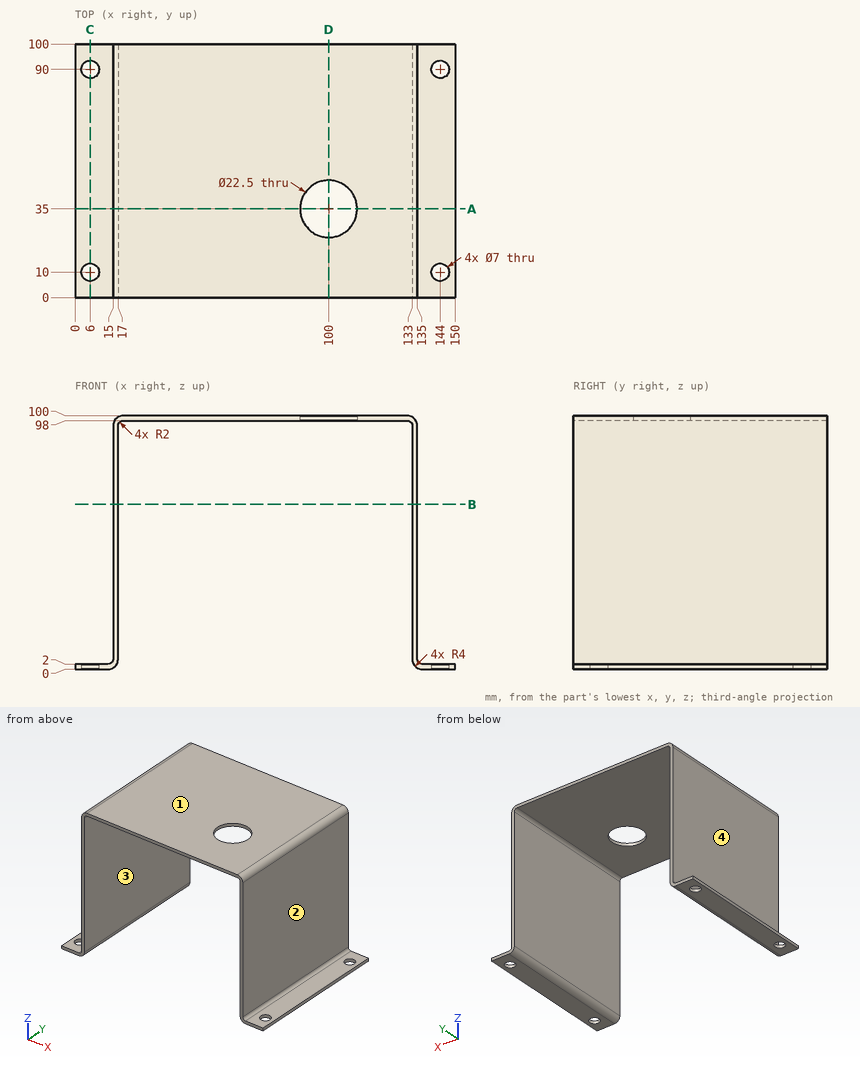
Could you check a few things on this drawing? It's one solid part, dimensions in mm from its lowest x, y, z. Coordinates: 2 decimals unless noted, no trailing zeros. Order: outer loops, then holes, each group sorted by start corner. A loop starts at its lowest first (then second) coordinate and runs counter-clockwise, first axis right, second up. Notation, with made-up numbers: M 27,43 L 47,43 A28 ccw 47,61 Z; hole C 88.5,0.25 d9. An arc over 180 degrees is marked long. Use one line per item in the form item = value. Start each with the question number.
1. Suppose I cut it at B-B on z = 65. Write out the boundary of the cut face in (x, y).
2. Please list where these lines run through material, in increasing order: line 1 (Y direction, x = 6, z = 0.5); line 2 (X direction, y = 78, z = 51); line 3 (X direction, y = 10, z = 1).
3. Suppose I cut it at D-D on x = 100. Write out the boundary of the cut face in (y, z), then the cut area to 3 significant figures.
4. For pin 1 (10.5 mm diameter, centred on x = 7.5, y = 60.5, fed in from +Z); pin 2 (6.5 mm diameter, centred on x = 6, y = 10, fed in from -Z) (3 decimals); pin 3 (8 mm diameter, centred on x = 50.5, y = 71, fed in from -Z); pin 4 (6 mm diameter, centred on y = 43.5, z = 54.5, fed in from +X), each with a flat end and sliding along its axis, tell me the tip position at first contact or that it passes through.
5. Suppose I cut it at A-A on y = 35. Write out the boundary of the cut face in (x, z).
6. We'd pull the mould along X, two halves only. Please class the marked faces 1, 2, 3 and 4: +X half, -X half, draft (parallel to the pull), parting line (faces both ways), or undercut.
7. Suppose I cut it at C-C on x = 6. Write out the boundary of the cut face in (y, z).
Geometry says:
q1.outline = M 15,0 L 17,0 L 17,100 L 15,100 Z; M 133,0 L 135,0 L 135,100 L 133,100 Z
q2.line_1 = 0 to 6.5, 13.5 to 86.5, 93.5 to 100
q2.line_2 = 15 to 17, 133 to 135
q2.line_3 = 0 to 2.5, 9.5 to 15.65, 134.35 to 140.5, 147.5 to 150
q3.outline = M 0,98 L 23.75,98 L 23.75,100 L 0,100 Z; M 46.25,98 L 100,98 L 100,100 L 46.25,100 Z
q3.area = 155 mm^2
q4.pin_1 = 2
q4.pin_2 = through
q4.pin_3 = 98
q4.pin_4 = 135
q5.outline = M 0,0 L 13,0 A4 ccw 17,4 L 17,96 A2 cw 19,98 L 88.75,98 L 88.75,100 L 19,100 A4 ccw 15,96 L 15,4 A2 cw 13,2 L 0,2 Z; M 111.25,98 L 131,98 A2 cw 133,96 L 133,4 A4 ccw 137,0 L 150,0 L 150,2 L 137,2 A2 cw 135,4 L 135,96 A4 ccw 131,100 L 111.25,100 Z
q6.face_1 = draft
q6.face_2 = +X half
q6.face_3 = undercut
q6.face_4 = -X half
q7.outline = M 0,0 L 6.5,0 L 6.5,2 L 0,2 Z; M 13.5,0 L 86.5,0 L 86.5,2 L 13.5,2 Z; M 93.5,0 L 100,0 L 100,2 L 93.5,2 Z
